Work out the finished part from the listing and answer in its coordinate system (mm). A direction names the side the tool comes from. Give positions to 0.01 mm unless a question says otherwise; leave off trailing zeros. Loops run counter-clockwise (first coordinate to the right, second up) from the corner with the lowest first, then second, coordinate; pieces in that order, holes last.
```python
from build123d import *

# Parameters (mm, degrees)
SKETCH1_R           = 250
SKETCH1_R_2         = 7.25
BOSS_EXTRUDE1_DEPTH = 9.5
SKETCH2_R           = 32
CUT_EXTRUDE1_DEPTH  = 8.5
SKETCH3_R           = 5
CUT_EXTRUDE2_DEPTH  = 355.063553617


with BuildPart() as part:
    # Sketch1 → Boss-Extrude1 (new, symmetric)
    with BuildSketch(Plane(origin=(0, 0, 0), x_dir=(1, 0, 0), z_dir=(0, 1, 0))):
        with Locations(Location((0, 0, 0), (0, 0, 270))):
            Circle(SKETCH1_R)
        with Locations(Location((0, 0, 0), (0, 0, 270))):
            Circle(SKETCH1_R_2, mode=Mode.SUBTRACT)
    extrude(amount=BOSS_EXTRUDE1_DEPTH, both=True)

    # Sketch2 → Cut-Extrude1 (cut)
    with BuildSketch(Plane(origin=(0, 9.5, 0), x_dir=(1, 0, 0), z_dir=(0, 1, 0))):
        with Locations(Location((0, 0, 0), (0, 0, 270))):
            Circle(SKETCH2_R)
    extrude(amount=-CUT_EXTRUDE1_DEPTH, mode=Mode.SUBTRACT)

    # Sketch3 → Cut-Extrude2 (cut, through all)
    with BuildSketch(Plane.XZ.offset(9.5)):
        with Locations(Location((111.25, 192.690652342, 0), (0, 0, 270))):
            Circle(SKETCH3_R)
        with Locations(Location((222.5, 0, 0), (0, 0, 270))):
            Circle(SKETCH3_R)
        with Locations(Location((-111.25, -192.690652342, 0), (0, 0, 90))):
            Circle(SKETCH3_R)
        with Locations(Location((-222.5, 0, 0), (0, 0, 90))):
            Circle(SKETCH3_R)
        with Locations(Location((-111.25, 192.690652342, 0), (0, 0, 270))):
            Circle(SKETCH3_R)
        with Locations(Location((111.25, -192.690652342, 0), (0, 0, 270))):
            Circle(SKETCH3_R)
    extrude(amount=-CUT_EXTRUDE2_DEPTH, mode=Mode.SUBTRACT)


solid = part.part
```
Q1. Which of the six approach directions +Z, -Z, +X, -X, +Y, -Y give full straight-line access (tool end or side, diameter ignored) to faces 1 (the face through (8, 1, 0)), 2 (the face through (-52, 9.5, -3))?
Q2. Given pin 1 (1 mm diameter, centred on y = -5.5, z = 58, fed in from -X); pin 2 (10 mm diameter, centred on x = 121.5, y = -4, fed in from +Z); pin 3 (10 mm diameter, centred on x = 182, y = 6, fed in from +Z), each flat-ended and moving along its own axis, determine where each tip first touches the part or whether it passes through.
Q3. Section D-D on z = 87 is taken. Give the vertices of the cut face in (x, y).
Q4. Determine the mould class of faces 3 (the face through (10.99, 0.13, -249.76)), 4 (the face through (-52, -9.5, -3)), 5 (the face through (-31.24, 5.31, -6.94)) for opening direction X: +X half, -X half, draft (parallel to the pull), parting line (faces both ways), or undercut.
Q5. Section A-A on x = 0 is taken. Give the vertices of the cut face in (y, z), plus the area to 3 significant figures.
Q6. Consider line 1 along Z through (x, y) = (-113, 3.5); line 2 along Z through (x, y) = (-21, 7.25); line 3 along Z through (x, y) = (218, 0.5). Determine where each line is inside the solid, lowest interval first.
Q7. Section C-C on x = -200 is taken. Give the vertices of the cut face in (y, z).
Q8. Section B-B on z = -19 is taken. Give the vertices of the cut face in (x, y), plus the area to 3 significant figures.
Check result:
1. face 1: +Y
1. face 2: +Z, -Z, +X, -X, +Y
2. pin 1: stops at x = -243.3
2. pin 2: stops at z = 221.2
2. pin 3: stops at z = 176.55
3. outline: (-234.37, -9.5) - (234.37, -9.5) - (234.37, 9.5) - (-234.37, 9.5) - close
4. face 3: parting line
4. face 4: draft
4. face 5: undercut
5. outline: (-9.5, -250) - (9.5, -250) - (9.5, -32) - (1, -32) - (1, -7.25) - (-9.5, -7.25) - close; (-9.5, 7.25) - (1, 7.25) - (1, 32) - (9.5, 32) - (9.5, 250) - (-9.5, 250) - close
5. area: 8,800 mm2
6. line 1: z = -223 to -197.37, -188.01 to 188.01, 197.37 to 223
6. line 2: z = -249.12 to -24.15, 24.15 to 249.12
6. line 3: z = -122.38 to -2.18, 2.18 to 122.38
7. outline: (-9.5, -150) - (9.5, -150) - (9.5, 150) - (-9.5, 150) - close
8. outline: (-249.28, -9.5) - (249.28, -9.5) - (249.28, 9.5) - (25.75, 9.5) - (25.75, 1) - (-25.75, 1) - (-25.75, 9.5) - (-249.28, 9.5) - close
8. area: 9,030 mm2
